Geometry check sheet. Reference: the model listing, model coordinates, mm. A direction names the side the tool comes from. Round coordinates to 2 decimals unless told otherwise and drop trailing zeros. Use a Markdown table: item, result.
```python
from build123d import *

# Parameters (mm, degrees)
SKETCH1_W               = 500
SKETCH1_H               = 30
BOSS_EXTRUDE1_DEPTH     = 15
CUT_EXTRUDE1_REACH      = 503.124
SKETCH2_W               = 35
SKETCH2_H               = 15
CUT_EXTRUDE2_DEPTH      = 502.796771612
CUT_EXTRUDE2_DEPTH_BACK = 502.796771612
SKETCH3_R               = 5
SKETCH3_R_2             = 7.5
FILLET3_R               = 15


with BuildPart() as part:
    # Sketch1 → Boss-Extrude1 (new, symmetric)
    with BuildSketch(Plane.XY):
        with Locations((250, 15)):
            Rectangle(SKETCH1_W, SKETCH1_H)
    extrude(amount=BOSS_EXTRUDE1_DEPTH, both=True)

    # Sketch2 → Cut-Extrude1 (cut, up to next)
    with BuildSketch(Plane(origin=(0, 30, 0), x_dir=(1, 0, 0), z_dir=(0, 1, 0)), mode=Mode.PRIVATE) as cut_extrude1_sk1:
        with Locations((17.5, 0)):
            Rectangle(SKETCH2_W, SKETCH2_H)
    cut_extrude1_tool1 = extrude(cut_extrude1_sk1.sketch, amount=-CUT_EXTRUDE1_REACH, mode=Mode.PRIVATE) & part.part
    add(cut_extrude1_tool1.solids().sort_by_distance((17.5, 30, 0))[0], mode=Mode.SUBTRACT)

    # Sketch3 → Cut-Extrude2 (cut, two sides: drawn at the far end of the back side and taken through both)
    with BuildSketch(Plane.XY.offset(15).offset(-CUT_EXTRUDE2_DEPTH_BACK)):
        with Locations((15, 15)):
            Circle(SKETCH3_R)
        with Locations((485, 15)):
            Circle(SKETCH3_R_2)
    extrude(amount=CUT_EXTRUDE2_DEPTH + CUT_EXTRUDE2_DEPTH_BACK, mode=Mode.SUBTRACT)

    # Fillet3
    fillet3_edges = [part.edges().sort_by_distance(p)[0] for p in [
        (500, 0, 0),
        (500, 30, 0),
        (0, 0, 11.25),
        (0, 0, -11.25),
        (0, 30, -11.25),
        (0, 30, 11.25),
    ]]
    fillet(fillet3_edges, radius=FILLET3_R - 0.0001)  # a hair under: the kernel refuses the full size


solid = part.part
```
(1) Access from +Z, -Z, +X, -X, +Y, -Y to the whole of each face (thin tool, end or side, straight path). Record for faces 5 (the face through (247, 30, 0)), 6 (the face through (35, 15, 0)).
A:
| item | result |
|---|---|
| face 5 | +Z, -Z, +X, -X, +Y |
| face 6 | -X, +Y, -Y |
(2) Gauge pin test, flat ends, axial feed: pin 1 Ø6 at (y, z) = (16, -3) entering from -X; pin 2 Ø12 at (y, z) = (8.5, -3) entering from -X; pin 3 Ø3 at (y, z) = (19.5, 12) entering from -X. Record the tip position at first contact, or that the pin passes through.
A:
| item | result |
|---|---|
| pin 1 | stops at x = 35 |
| pin 2 | stops at x = 0.22 |
| pin 3 | stops at x = 0.3 |
(3) Thickness scan on line 1 (X direction, y = 15, z = 11); line 2 (X direction, y = 14.5, z = -3.25); line 3 (Y direction, x = 15, z = -11.25). Record the ranges inside material, lowest first.
A:
| item | result |
|---|---|
| line 1 | x = 0 to 10, 20 to 477.5, 492.5 to 500 |
| line 2 | x = 35 to 477.52, 492.48 to 499.99 |
| line 3 | y = 0 to 10, 20 to 30 |
(4) Release check for a two-part mould opening along X. For faces 1 (the face through (247, 15, -15)), 2 (the face through (491.93, 12.13, -0.21)), 3 (the face through (495.49, 4.28, 0.21)), 4 (the face through (4.51, 4.28, 11.3)) record: +X half, -X half, draft (parallel to the pull), parting line (faces both ways), or undercut.
A:
| item | result |
|---|---|
| face 1 | draft |
| face 2 | undercut |
| face 3 | +X half |
| face 4 | -X half |
